Build history of the part. All positions in model axes, mm. Face numbers are marked on the shaded views. Round coordinates to 2 decimals unless told otherwise and drop trailing zeros. Write each loop counter-clockwise with the first axis right and the second up, starting at its lowest first coordinate (ties: lowest second). Pieces come first, ordered by that corner, then holes.
from build123d import *

# Parameters (mm, degrees)
F0_R           = 10
F0_R_2         = 6.1
F1_DEPTH       = 6
F2_DEPTH       = 10
F4_R           = 1
F1_FACE_R      = 10
F7_D           = 4.2
F7_CBORE_D     = 7
F7_CBORE_DEPTH = 4
F8_D           = 3.2
F8_DEPTH       = 8
F8_START       = 6
F8_TIP         = 0.9613769904
F6_R           = 10
F10_DEPTH      = 8
F12_DEPTH      = 10


with BuildPart() as f1:
    # F0 (on Top) → F1 (new body)
    with BuildSketch(Plane.XY):
        Circle(F0_R)
        Circle(F0_R_2, mode=Mode.SUBTRACT)
        Circle(F0_R_2)
    extrude(amount=F1_DEPTH)

    # F0 (on Top) → F2 (join)
    with BuildSketch(Plane.XY):
        Circle(F0_R)
        Circle(F0_R_2, mode=Mode.SUBTRACT)
    extrude(amount=-F2_DEPTH)

    # F7 (through all)
    with Locations(Plane(origin=(0, 0, 0), x_dir=(1, 0, 0), z_dir=(0, 0, -1))):
        with Locations((0, 0)):
            CounterBoreHole(F7_D / 2, F7_CBORE_D / 2, F7_CBORE_DEPTH)


with BuildPart() as f5:
    # F4 (on offset) → F5 section 0
    with BuildSketch(Plane.XY.offset(16)):
        Circle(F4_R)
    # F1_face (on face) → F5 section 1
    with BuildSketch(Plane.XY.offset(6)):
        Circle(F1_FACE_R)
    loft()

    # F8
    # its depths count from where the whole tool has entered the part; down to there all is cleared
    with Locations(Plane(origin=(0, 0, 0), x_dir=(1, 0, 0), z_dir=(0, 0, -1)).offset(-F8_START)):
        with Locations((0, 0)):
            Hole(F8_D / 2, depth=F8_DEPTH)
            with Locations((0, 0, -(F8_DEPTH + F8_TIP / 2))):  # 118° drill point
                Cone(0, F8_D / 2, F8_TIP, mode=Mode.SUBTRACT)

    # F6 (on face) → F10 (join)
    with BuildSketch(Plane.XY.offset(6)):
        Circle(F6_R)
    extrude(amount=-F10_DEPTH)

    # F11 (on face) → F12 (cut)
    with BuildSketch(Plane(origin=(0, 0, -2), x_dir=(1, 0, 0), z_dir=(0, 0, -1))):
        with BuildLine():
            ThreePointArc((1.6, 0), (0, 1.6), (-1.6, 0))
            ThreePointArc((-1.6, 0), (0, -1.6), (1.6, 0))
        make_face()
    extrude(amount=-F12_DEPTH, mode=Mode.SUBTRACT)


solid = f5.part
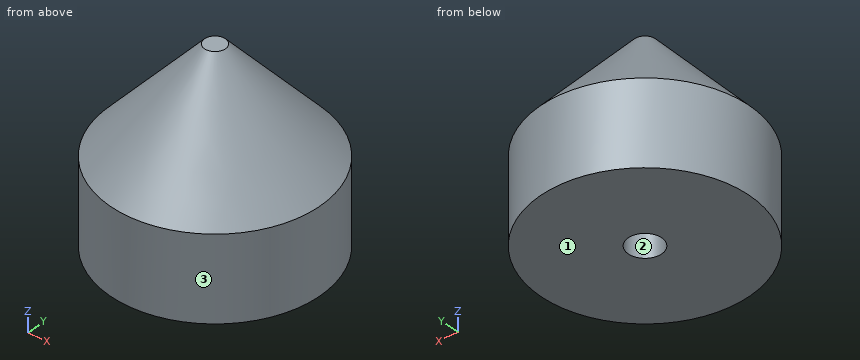
1) Wall check: L1, parallel to Y at x = 0, z = 3; L2, parallel to Y at x = 0, z = 7.75 (3 decimals); L3, parallel to Z at x = -4.75, y = -5.75. Give the ranges that are in metal, low to high.
Results:
L1: y = -10 to -1.6, 1.6 to 10
L2: y = -8.425 to -1.6, 1.6 to 8.425
L3: z = -2 to 8.82
2) Slice it at A-A (z = 10.5). Write the cut outline in (x, y), plus the area to 3 significant figures.
Results:
outline: circle Ø11.9 at (0, 0); hole circle Ø3.2 at (0, 0)
area: 103 mm2
3) Mould opens along Y. For the marked faces 1, 2 and 3 say: released by +Y, released by -Y, zero draft, split by the parting line, or undercut.
Results:
face 1: zero draft
face 2: undercut
face 3: split by the parting line
4) Slice it at B-B (z = 0.25). Write the cut outline in (x, y), plus the area to 3 significant figures.
Results:
outline: circle Ø20 at (0, 0); hole circle Ø3.2 at (0, 0)
area: 306 mm2
5) Pin check, flat tips, straight feed: pin 1 Ø3 at (x, z) = (4, 11.5) entering from -Y; pin 2 Ø6 at (x, z) = (-0.5, 14) entering from -Y; pin 3 Ø8 at (x, z) = (6, 7.5) entering from -Y; pin 4 Ø10 at (x, z) = (-4.5, 3.5) entering from +Y. Stop position of each tip, or through.
Results:
pin 1: stops at y = -5.3
pin 2: stops at y = -5.49
pin 3: stops at y = -9.73
pin 4: stops at y = 10
